The model under review builds one solid part; all positions refer to its coordinate system, in mm. Face numbers are marked on the shaded views. A direction names the side the tool comes from. Round coordinates to 2 decimals unless told otherwise and drop trailing zeros. Order: outer loops, then holes, each group sorted by start corner. A loop starts at its lowest first (then second) coordinate and runs counter-clockwise, first axis right, second up. Notation, with made-up numbers: (43.25, 47.5) -> (71.25, 47.5) arc R13 ccw to (71.25, 65.5) -> close; hole circle Ø8 at (41, 47.5). An arc over 180 degrees is marked (long way). Return JSON: item names as keys, results as strings. Group by question number.
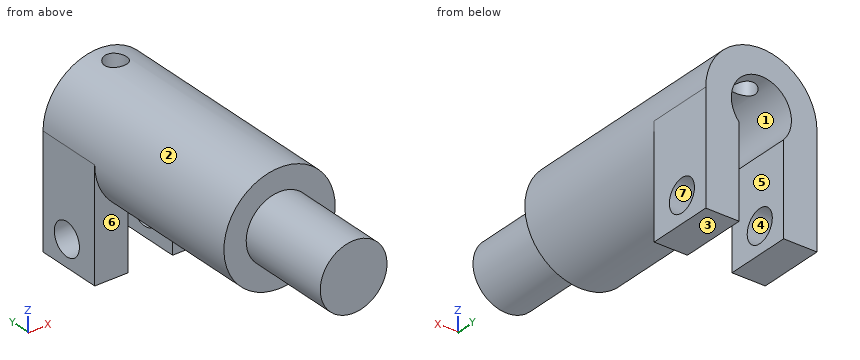
from build123d import *

# Parameters (mm, degrees)
SKETCH1_R                   = 6.35
SKETCH1_R_2                 = 3.429
BOSS_EXTRUDE1_DEPTH         = 19.05
SKETCH2_R                   = 3.81
BOSS_EXTRUDE2_DEPTH         = 10.922
SKETCH3_R                   = 3.429
BOSS_EXTRUDE3_DEPTH         = 7.62
M3_CLEARANCE_HOLE1_D        = 3.7
M3_CLEARANCE_HOLE1_DEPTH    = 25.4
M3_CLEARANCE_HOLE1_TIP      = 1.111592145
CUT_EXTRUDE1_START          = -8.89
CUT_EXTRUDE1_DEPTH          = 8.89
TAP_DRILL_FOR_M3X0_5_TAP1_D = 2.5


with BuildPart() as part:
    # Sketch1 → Boss-Extrude1 (new body)
    with BuildSketch(Plane(origin=(0, 0, 0), x_dir=(1, 0, 0), z_dir=(0, 1, 0))):
        with Locations(Location((0, 0, 0), (0, 0, 90))):
            Circle(SKETCH1_R)
        with Locations(Location((0, 0, 0), (0, 0, 90))):
            Circle(SKETCH1_R_2, mode=Mode.SUBTRACT)
    extrude(amount=BOSS_EXTRUDE1_DEPTH)

    # Sketch2 → Boss-Extrude2 (add)
    with BuildSketch(Plane.XZ):
        with Locations(Location((0, 0, 0), (0, 0, 90))):
            Circle(SKETCH2_R)
    extrude(amount=BOSS_EXTRUDE2_DEPTH)

    # Sketch3 → Boss-Extrude3 (add)
    with BuildSketch(Plane(origin=(0, 19.05, 0), x_dir=(1, 0, 0), z_dir=(0, 1, 0))):
        with BuildLine():
            Line((2.54, 12.7), (2.54, 5.819871133))
            ThreePointArc((2.54, 5.819871133), (0, 6.35), (-2.54, 5.819871133))
            Line((-2.54, 5.819871133), (-2.54, 12.7))
            Line((-2.54, 12.7), (-6.35, 12.7))
            Line((-6.35, 12.7), (-6.35, 0))
            ThreePointArc((-6.35, 0), (0, -6.35), (6.35, 0))
            Line((6.35, 0), (6.35, 12.7))
            Line((6.35, 12.7), (2.54, 12.7))
        make_face()
        with Locations(Location((0, 0, 0), (0, 0, 90))):
            Circle(SKETCH3_R, mode=Mode.SUBTRACT)
    extrude(amount=BOSS_EXTRUDE3_DEPTH)

    # M3 Clearance Hole1
    with Locations(Plane.ZY.offset(6.35)):
        with Locations((-9.714139502, 23.151538797)):
            Hole(M3_CLEARANCE_HOLE1_D / 2, depth=M3_CLEARANCE_HOLE1_DEPTH)
            with Locations((0, 0, -(M3_CLEARANCE_HOLE1_DEPTH + M3_CLEARANCE_HOLE1_TIP / 2))):  # 118° drill point
                Cone(0, M3_CLEARANCE_HOLE1_D / 2, M3_CLEARANCE_HOLE1_TIP, mode=Mode.SUBTRACT)

    # Sketch7 → Cut-Extrude1 (cut)
    with BuildSketch(Plane(origin=(0, 26.67, 0), x_dir=(1, 0, 0), z_dir=(0, 1, 0)).offset(CUT_EXTRUDE1_START)):
        with BuildLine():
            Line((2.54, 2.303571358), (2.54, 5.819871133))
            ThreePointArc((2.54, 5.819871133), (0, 6.35), (-2.54, 5.819871133))
            Line((-2.54, 5.819871133), (-2.54, 2.303571358))
            ThreePointArc((-2.54, 2.303571358), (0, 3.429), (2.54, 2.303571358))
        make_face()
    extrude(amount=CUT_EXTRUDE1_DEPTH, mode=Mode.SUBTRACT)

    # Tap Drill for M3x0.5 Tap1 (through all)
    with Locations(Plane(origin=(-0.033798391, 24.130572857, 6.349910052), x_dir=(0.999985834964, 0, 0.005322581268), z_dir=(-0.005322581268, 0, 0.999985834964))):
        with Locations((0, 0)):
            Hole(TAP_DRILL_FOR_M3X0_5_TAP1_D / 2)


solid = part.part
Item 1: Consider section A-A on z = -7. State the section outline as (x, y) points.
Item 2: Consider section B-B on y = 22.5. State the section outline as (x, z) points, plus the area to 3 significant figures.
Item 3: For the marked faces 1, 2 and 3, list the 3-axis set-ups (+Z, -Z, +X, -X, +Y, -Y) from which the entire face can be reached by the end or side of a thin tool; tool diameter is ignored.
Item 4: Wall thickness on line 1 along X through (y, z) = (24.5, -6); line 2 along Y through (x, z) = (4.5, 3.5); line 3 along Y through (x, z) = (4, -5): over which ranges is each line inside the solid? List them lowest first.
Item 5: Consider section D-D on z = -9.25. State the section outline as (x, y) points, plus the area to 3 significant figures.
Item 6: The part is to be moulded in two halves that separate along Y. For the marked faces 4, 5, 6 and 7, say which applies: +Y half, -Y half, draft (parallel to the pull), parting line (faces both ways), or undercut.
Item 7: Consider section C-C on x = -4.25. State the section outline as (y, z) points.
Item 8: Insertion check: pin 1 Ø4 at (y, z) = (-3, -2.5) entering from -X; pin 2 Ø2 at (x, z) = (0.5, -5) entering from +Y; pin 3 Ø3 at (x, z) = (-3.5, -7.5) entering from -Y. Each pin has a flat end and moves straight along its axis. Give the tip position at first contact, or say it passes through.
Values:
{
 "1": {"outline": "(-6.35, 19.05) -> (-2.54, 19.05) -> (-2.54, 26.67) -> (-6.35, 26.67) -> close; (2.54, 19.05) -> (6.35, 19.05) -> (6.35, 26.67) -> (2.54, 26.67) -> close"},
 "2": {"outline": "(-6.35, -12.7) -> (-2.54, -12.7) -> (-2.54, -11.45) -> (-6.35, -11.45) -> close; (-6.35, -7.98) -> (-2.54, -7.98) -> (-2.54, -2.3) arc R3.43 cw (long way) to (2.54, -2.3) -> (2.54, -7.98) -> (6.35, -7.98) -> (6.35, 0) arc R6.35 ccw to (-6.35, 0) -> close; (2.54, -12.7) -> (6.35, -12.7) -> (6.35, -11.45) -> (2.54, -11.45) -> close", "area": "112 mm^2"},
 "3": {"face 1": "+Y", "face 2": "-Y", "face 3": "-Z, +X, -X, +Y, -Y"},
 "4": {"line 1": "-6.35 to -2.54, 2.54 to 6.35", "line 2": "0 to 26.67", "line 3": "19.05 to 26.67"},
 "5": {"outline": "(-6.35, 19.05) -> (-2.54, 19.05) -> (-2.54, 21.36) -> (-6.35, 21.36) -> close; (-6.35, 24.94) -> (-2.54, 24.94) -> (-2.54, 26.67) -> (-6.35, 26.67) -> close; (2.54, 19.05) -> (6.35, 19.05) -> (6.35, 21.36) -> (2.54, 21.36) -> close; (2.54, 24.94) -> (6.35, 24.94) -> (6.35, 26.67) -> (2.54, 26.67) -> close", "area": "30.8 mm^2"},
 "6": {"face 4": "undercut", "face 5": "draft", "face 6": "-Y half", "face 7": "undercut"},
 "7": {"outline": "(0, -4.72) -> (19.05, -4.72) -> (19.05, -12.7) -> (26.67, -12.7) -> (26.67, 4.72) -> (0, 4.72) -> close; hole circle Ø3.7 at (23.15, -9.71)"},
 "8": {"pin 1": "x = -3.78", "pin 2": "y = 17.78", "pin 3": "y = 19.05"}
}
